```python
from build123d import *

# Parameters (mm, degrees)
F1_DEPTH = 1
F2_DEPTH = 3
F3_DEPTH = 2


with BuildPart() as f1:
    # F0 (on Right) → F1 (new body)
    with BuildSketch(Plane.YZ):
        Polygon((-35.161479, 26.232064), (-35.161479, 53.232064), (-81.161479, 53.232064), (-73.265584, 46.433675), (-62.346259, 26.232064), (-55.265479, 13.132064), (-52.265479, 13.132064), (-52.265479, 26.232064), (-45.161479, 26.232064), align=None)
    extrude(amount=F1_DEPTH)

    # F0 (on Right) → F2 (join)
    with BuildSketch(Plane.YZ):
        Polygon((-73.265584, 46.433675), (-81.161479, 53.232064), (-81.161479, 51.912471), (-74.057687, 45.796085), (-56.402211, 13.132064), (-55.265479, 13.132064), (-62.346259, 26.232064), align=None)
    extrude(amount=F2_DEPTH)

    # F0 (on Right) → F3 (join)
    with BuildSketch(Plane.YZ):
        Polygon((-74.057687, 45.796085), (-81.161479, 51.912471), (-81.161479, 26.232064), (-81.161479, 13.132064), (-56.402211, 13.132064), align=None)
    extrude(amount=F3_DEPTH)


solid = f1.part
```
Could you check a few things on this model? Use its own coordinates, in mm. A direction names the side the tool comes from. Round coordinates to 2 decimals unless told otherwise and drop trailing zeros. Write each loop counter-clockwise with the first axis right and the second up, starting at its lowest first coordinate (ties: lowest second). Pieces come first, ordered by that corner, then holes. Notation, with made-up numbers: M 23.5,24 L 67.5,24 A19 ccw 67.5,35 Z; hole C 6.5,78 d1. An arc over 180 degrees is marked long. Answer in a Markdown table with one row per item. Add a question column.
Q1. Imagine slicing it at A-A (y = -72). Please give me the cut outline in (x, z).
Q2. On a 3-axis mill with a long thin cutter (end or side, diameter ignored), from which of +Z, -Z, +X, -X, +Y, -Y can I reach the whole of each face in a straight line? I mean faces 1 (the flat face through (1, -53, 38)), 2 (the flat face through (0, -58, 33)), 3 (the flat face through (0.5, -57.8, 53.232)), 4 (the flat face through (2.49, -65.35, 29.69)), 5 (the flat face through (0.5, -43.8, 26.232)). Say none if no direction works.
Q3. Imagine slicing it at C-C (y = -46). Please give me the cut outline in (x, z).
Q4. Imagine slicing it at B-B (z = 34). Please give me the cut outline in (x, y).
Q5. If I drill on line 1 (X direction, y = -41, z = 35); line 2 (X direction, y = -65.5, z = 21.5); line 3 (Y direction, x = 0.6, z = 22.5), over which ranges is the centre line in solid material (lowest first)? Write a range as from..to.
Q6. Will these pins go through, and if not, where does the flat tip stop? pin 1 Ø0.8 at (x, y) = (0.5, -39.5) entering from -Z; pin 2 Ø0.5 at (x, z) = (0.5, 21.5) entering from +Y.
Values:
| question | item | result |
|---|---|---|
| 1 | outline | M 0,13.13 L 2,13.13 L 2,41.99 L 3,41.99 L 3,44.09 L 1,44.09 L 1,53.23 L 0,53.23 Z |
| 2 | face 1 | +Z, +X, +Y |
| 2 | face 2 | +Z, -Z, -X, +Y, -Y |
| 2 | face 3 | +Z, +X, -X, +Y, -Y |
| 2 | face 4 | -Z, +X, -Y |
| 2 | face 5 | -Z, +X, -X, +Y |
| 3 | outline | M 0,26.23 L 1,26.23 L 1,53.23 L 0,53.23 Z |
| 4 | outline | M 0,-81.16 L 2,-81.16 L 2,-67.68 L 3,-67.68 L 3,-66.54 L 1,-66.54 L 1,-35.16 L 0,-35.16 Z |
| 5 | line 1 | 0..1 |
| 5 | line 2 | 0..2 |
| 5 | line 3 | -81.16..-52.27 |
| 6 | pin 1 | z = 26.23 |
| 6 | pin 2 | y = -52.27 |
